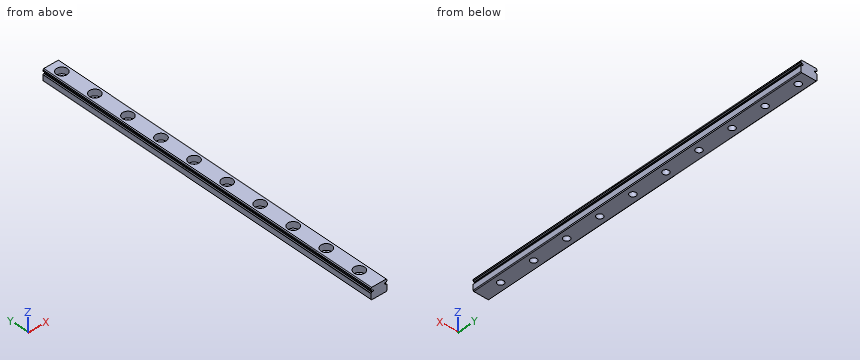
```python
from build123d import *

# Parameters (mm, degrees)
RESSALTO_EXTRUS_O1_DEPTH                             = 1000
CORTE_EXTRUS_O1_START                                = -1000
CORTE_EXTRUS_O1_DEPTH                                = 1000
CORTE_EXTRUS_O2_DEPTH                                = 1001.031261626
CORTE_EXTRUS_O3_DEPTH                                = 1001.031261626
CORTE_EXTRUS_O4_DEPTH                                = 1001.031261626
CORTE_EXTRUS_O5_DEPTH                                = 0.002166667
CORTE_EXTRUS_O6_DEPTH                                = 0.002166667
CORTE_EXTRUS_O7_DEPTH                                = 0.002166667
CORTE_EXTRUS_O8_DEPTH                                = 0.002166667
INCLINA_O1_ANGLE                                     = 45.1469538
ESBO_O10_W                                           = 0.450000001
ESBO_O10_H                                           = 1000
REBAIXO_PARA_PARAFUSO_DE_M_QUINA_DE_CABE_D           = 3.5
REBAIXO_PARA_PARAFUSO_DE_M_QUINA_DE_CABE_CBORE_D     = 6
REBAIXO_PARA_PARAFUSO_DE_M_QUINA_DE_CABE_CBORE_DEPTH = 3.50000002
CHANFRO1_SIZE                                        = 0.062563219
CHANFRO1_SIZE2                                       = 0.062205617
CHANFRO3_START                                       = -3.730761794
CHANFRO3_DEPTH                                       = 0.399013115
CHANFRO4_SIZE                                        = 0.4
FILETE1_R                                            = 0.130000023
SKETCH1_W                                            = 36.072768502
SKETCH1_H                                            = 801.847062841
SKETCH1_W_2                                          = 21.632087489
SKETCH1_H_2                                          = 62.411000867
CUT_EXTRUDE1_DEPTH                                   = 10


with BuildPart() as part:
    # Esboço1 → Ressalto-extrusão1 (new body)
    with BuildSketch(Plane.XZ):
        with BuildLine():
            Line((4.5, 5.4097155), (4.5, 6.01167813))
            Line((4.5, 6.01167813), (4.1, 6.50000002))
            Line((4.1, 6.50000002), (-4.1, 6.50000002))
            Line((-4.1, 6.50000002), (-4.5, 6.01167813))
            Line((-4.5, 6.01167813), (-4.5, 2e-08))
            Line((-4.5, 2e-08), (4.5, 2e-08))
            Line((4.5, 2e-08), (4.5, 3.50196265))
            ThreePointArc((4.5, 3.50196265), (4.477413879, 3.553810372), (4.43494978, 3.59116167))
            ThreePointArc((4.43494978, 3.59116167), (3.930462682, 4.43021964), (4.43494978, 5.26927761))
            ThreePointArc((4.43494978, 5.26927761), (4.490651601, 5.328761203), (4.5, 5.4097155))
        make_face()
    extrude(amount=-RESSALTO_EXTRUS_O1_DEPTH)

    # Esboço2 → Corte-extrusão1 (cut)
    with BuildSketch(Plane(origin=(0, 1000, 0), x_dir=(-1, 0, 0), z_dir=(0, 1, 0)).offset(CORTE_EXTRUS_O1_START)):
        with BuildLine():
            Line((-4.030498711, 4.00588336), (-3.673447948, 4.00588336))
            ThreePointArc((-3.673447948, 4.00588336), (-3.223447946, 4.455883362), (-3.673447948, 4.905883363))
            Line((-3.673447948, 4.905883363), (-3.953580008, 4.905883363))
            ThreePointArc((-3.953580008, 4.905883363), (-4.010719931, 4.899199784), (-4.065149208, 4.917830263))
            ThreePointArc((-4.065149208, 4.917830263), (-3.93114763, 4.466290066), (-4.030498711, 4.00588336))
        make_face()
    extrude(amount=CORTE_EXTRUS_O1_DEPTH, mode=Mode.SUBTRACT)

    # Esboço3 → Corte-extrusão2 (cut, through all)
    with BuildSketch(Plane(origin=(0, 1000, 0), x_dir=(-1, 0, 0), z_dir=(0, 1, 0))):
        with BuildLine():
            Line((4.5, 4.03150278), (4.5, 4.88017535))
            Line((4.5, 4.88017535), (3.66946318, 4.88017535))
            ThreePointArc((3.66946318, 4.88017535), (3.969667593, 4.455839065), (3.66946318, 4.03150278))
            Line((3.66946318, 4.03150278), (4.5, 4.03150278))
        make_face()
    extrude(amount=-CORTE_EXTRUS_O2_DEPTH, mode=Mode.SUBTRACT)

    # Esboço4 → Corte-extrusão3 (cut, through all)
    with BuildSketch(Plane(origin=(0, 1000, 0), x_dir=(-1, 0, 0), z_dir=(0, 1, 0))):
        with BuildLine():
            Line((4.026513974, 4.88017535), (4.5, 4.88017535))
            Line((4.5, 4.88017535), (4.5, 5.328056964))
            ThreePointArc((4.5, 5.328056964), (4.223646078, 5.145991535), (4.026513974, 4.88017535))
        make_face()
    extrude(amount=-CORTE_EXTRUS_O3_DEPTH, mode=Mode.SUBTRACT)

    # Esboço5 → Corte-extrusão4 (cut, through all)
    with BuildSketch(Plane(origin=(0, 1000, 0), x_dir=(-1, 0, 0), z_dir=(0, 1, 0))):
        with BuildLine():
            Line((4.5, 3.583620931), (4.5, 4.03150278))
            Line((4.5, 4.03150278), (4.026513856, 4.03150278))
            ThreePointArc((4.026513856, 4.03150278), (4.223645982, 3.76568645), (4.5, 3.583620931))
        make_face()
    extrude(amount=-CORTE_EXTRUS_O4_DEPTH, mode=Mode.SUBTRACT)

    # Esboço6 → Corte-extrusão5 (cut)
    with BuildSketch(Plane(origin=(0, 1000, 0), x_dir=(-1, 0, 0), z_dir=(0, 1, 0))):
        Polygon((0.891369267, 3.403698133), (0.714701433, 3.168235633), (0.2187042, 2.61105), (1.0945792, 2.61105), (1.0945792, 2.695983333), (0.398689633, 2.695983333), (0.794326433, 3.149466667), (0.9743123, 3.3891), (1.067110588, 3.573407857), (0.95413722, 3.802321701), (0.7876908, 3.88505), (0.54301, 3.88505), (0.375434678, 3.803592619), (0.295011167, 3.6384023), (0.295011167, 3.562), (0.3812718, 3.562), (0.3812718, 3.631766667), (0.437672733, 3.743620833), (0.549645633, 3.800116667), (0.7802262, 3.800116667), (0.893028067, 3.743810633), (0.976240026, 3.576039029), align=None)
    extrude(amount=-CORTE_EXTRUS_O5_DEPTH, mode=Mode.SUBTRACT)

    # Esboço7 → Corte-extrusão6 (cut)
    with BuildSketch(Plane.XZ):
        Polygon((-0.214632167, 3.88505), (-0.953983333, 3.88505), (-0.953983333, 2.61105), (-0.214632167, 2.61105), (-0.214632167, 2.695983333), (-0.86905, 2.695983333), (-0.86905, 3.205583333), (-0.5123963, 3.205583333), (-0.5123963, 3.290516667), (-0.86905, 3.290516667), (-0.86905, 3.800116667), (-0.214632167, 3.800116667), align=None)
    extrude(amount=-CORTE_EXTRUS_O6_DEPTH, mode=Mode.SUBTRACT)

    # Esboço8 → Corte-extrusão7 (cut)
    with BuildSketch(Plane(origin=(0, 1000, 0), x_dir=(-1, 0, 0), z_dir=(0, 1, 0))):
        Polygon((-0.214632167, 3.88505), (-0.953983333, 3.88505), (-0.953983333, 2.61105), (-0.214632167, 2.61105), (-0.214632167, 2.695983333), (-0.86905, 2.695983333), (-0.86905, 3.205583333), (-0.5123963, 3.205583333), (-0.5123963, 3.290516667), (-0.86905, 3.290516667), (-0.86905, 3.800116667), (-0.214632167, 3.800116667), align=None)
    extrude(amount=-CORTE_EXTRUS_O7_DEPTH, mode=Mode.SUBTRACT)

    # Esboço9 → Corte-extrusão8 (cut)
    with BuildSketch(Plane.XZ):
        Polygon((0.510057167, 3.620830633), (0.6071, 3.718655633), (0.6071, 2.609403333), (0.692033333, 2.609403333), (0.692033333, 3.883403333), (0.6741176, 3.883403333), (0.6741176, 3.795069794), (0.3690544, 3.640736667), (0.3690544, 3.551253333), align=None)
    extrude(amount=-CORTE_EXTRUS_O8_DEPTH, mode=Mode.SUBTRACT)

    # Inclinação1
    inclina_o1_faces = [part.faces().sort_by_distance(p)[0] for p in [
        (0.6741176, 0.001083333, 3.839236564),
    ]]
    draft(inclina_o1_faces, Plane(origin=(0.692033333, 0.002166667, 3.883403333), x_dir=(-1, 0, 0), z_dir=(0, 0, -1)), INCLINA_O1_ANGLE)

    # Esboço10 → Corte-Revolução1 (revolve, cut)
    with BuildSketch(Plane.XY.offset(4.455839065)):
        with Locations((-3.294667591, 500)):
            Rectangle(ESBO_O10_W, ESBO_O10_H)
    revolve(axis=Axis((-3.519667591, 1000, 4.455839065), (0, -1, 0)), mode=Mode.SUBTRACT)

    # Rebaixo para parafuso de máquina de cabeça sextavada de M31 (through all)
    with Locations(Plane.XY.offset(6.50000002)):
        with Locations((0, 990), (0, 970), (0, 950), (0, 930), (0, 910), (0, 890), (0, 870), (0, 850), (0, 830), (0, 810), (0, 790), (0, 770), (0, 750), (0, 730), (0, 710), (0, 690), (0, 670), (0, 650), (0, 630), (0, 610), (0, 590), (0, 570), (0, 550), (0, 530), (0, 510), (0, 490), (0, 470), (0, 450), (0, 430), (0, 410), (0, 390), (0, 370), (0, 350), (0, 330), (0, 310), (0, 290), (0, 270), (0, 250), (0, 230), (0, 210), (0, 190), (0, 170), (0, 150), (0, 130), (0, 110), (0, 90), (0, 70), (0, 50), (0, 30), (0, 10)):
            CounterBoreHole(REBAIXO_PARA_PARAFUSO_DE_M_QUINA_DE_CABE_D / 2, REBAIXO_PARA_PARAFUSO_DE_M_QUINA_DE_CABE_CBORE_D / 2, REBAIXO_PARA_PARAFUSO_DE_M_QUINA_DE_CABE_CBORE_DEPTH)

    # Chanfro1
    chanfro1_edges = [part.edges().sort_by_distance(p)[0] for p in [
        (-0.976240026, 999.998916667, 3.576039029),
    ]]
    chanfro1_side = [part.faces().sort_by_distance(p)[0] for p in [
        (-0.933804646, 999.998916667, 3.489868581),
    ]]
    chamfer(chanfro1_edges, length=CHANFRO1_SIZE, length2=CHANFRO1_SIZE2, reference=chanfro1_side[0])

    # Chanfro3: read off the stored shape, not the designer's step
    # Chanfro3 outline → Chanfro3 (add)
    with BuildSketch(Plane(origin=(0, 0, 0), x_dir=(0.8991051825477068, 0, 0.43773264753254887), z_dir=(0.4377326475325489, 0, -0.8991051825477069)).offset(CHANFRO3_START)):
        Polygon((1.327401403, -999.997833333), (1.31122788, -999.997833333), (1.311999664, -1000), (1.327401403, -1000), align=None)
    extrude(amount=CHANFRO3_DEPTH)

    # Chanfro4
    chanfro4_edges = [part.edges().sort_by_distance(p)[0] for p in [
        (4.5, 500, 2e-08),
        (-4.5, 500, 2e-08),
    ]]
    chamfer(chanfro4_edges, length=CHANFRO4_SIZE)

    # Filete1
    filete1_edges = [part.edges().sort_by_distance(p)[0] for p in [
        (4.030498711, 500, 4.00588336),
        (-4.026513974, 500, 4.88017535),
        (-4.5, 500, 5.328056964),
        (-4.5, 500, 3.583620931),
        (-4.026513856, 500, 4.03150278),
    ]]
    fillet(filete1_edges, radius=FILETE1_R)

    # Sketch1 → Cut-Extrude1 (cut)
    with BuildSketch(Plane(origin=(0, 0, 0), x_dir=(-1, 0, 0), z_dir=(0, 0, -1))):
        with Locations((-9.39117436, 617.429605919)):
            Rectangle(SKETCH1_W, SKETCH1_H)
        with Locations((0.25600221, -13.052857141)):
            Rectangle(SKETCH1_W_2, SKETCH1_H_2)
    extrude(amount=-CUT_EXTRUDE1_DEPTH, mode=Mode.SUBTRACT)


solid = part.part
```
Could you check a few things on this model? Use its own coordinates, in mm. Coordinates: 2 decimals unless noted, no trailing zeros. Loops run counter-clockwise (first coordinate to the right, second up) from the corner with the lowest first, then second, coordinate; pieces in that order, holes last.
1) Please list where these lines run through material, in increasing order: line 1 along Z through (x, y) = (4, 123); line 2 along X through (y, z) = (150, 1.95); line 3 along X through (y, z) = (92, 5).
Reported:
line 1: z = 0 to 4, 4.9 to 6.5
line 2: x = -4.5 to -1.75, 1.75 to 4.5
line 3: x = -4.1 to -2.24, 2.24 to 4.12
2) Will these pins go through, and if not, where does the flat tip stop? pin 1 Ø5 at (x, y) = (0, 110) entering from +Z; pin 2 Ø2.5 at (y, z) = (102, 1) entering from +X.
Reported:
pin 1: stops at z = 3
pin 2: stops at x = 4.5
3) Imagine slicing it at B-B (x = 0). State how many separate pieces and enclosed holes the cut face has, and give its area (3 significant figures).
Reported:
separate pieces: 11
enclosed holes: 0
area: 974 mm2
4) Imagine slicing it at A-A (y = 58.5). List the corners of the cut face in (x, z) for me.
Reported:
outline: (-4.5, 0.4) - (-4.1, 0) - (4.1, 0) - (4.5, 0.4) - (4.5, 3.5) arc R0.13 ccw to (4.43, 3.59) arc R0.95 cw to (4.07, 3.94) arc R0.13 ccw to (3.95, 4.01) - (3.67, 4.01) arc R0.45 cw to (3.67, 4.91) - (3.95, 4.91) arc R0.13 ccw to (4.07, 4.92) arc R0.95 cw to (4.43, 5.27) arc R0.13 ccw to (4.5, 5.41) - (4.5, 6.01) - (4.1, 6.5) - (-4.1, 6.5) - (-4.5, 6.01) - (-4.5, 5.41) arc R0.13 ccw to (-4.43, 5.29) arc R0.95 cw to (-4.06, 4.94) arc R0.13 ccw to (-3.95, 4.88) - (-3.67, 4.88) arc R0.45 cw (long way) to (-3.67, 4.03) - (-3.95, 4.03) arc R0.13 ccw to (-4.06, 3.97) arc R0.95 cw to (-4.43, 3.62) arc R0.13 ccw to (-4.5, 3.5) - close
